```python
from build123d import *

# Parameters (mm, degrees)
SKETCH1_W           = 12.7
SKETCH1_H           = 152.4
BOSS_EXTRUDE1_DEPTH = 25.4
SKETCH6_W           = 50.8
SKETCH6_H           = 25.4
BOSS_EXTRUDE5_DEPTH = 2.54
SKETCH7_W           = 2.54
SKETCH7_H           = 25.4
BOSS_EXTRUDE6_DEPTH = 25.4


with BuildPart() as part:
    # Sketch1 → Boss-Extrude1 (new body)
    with BuildSketch(Plane(origin=(0, 0, 0), x_dir=(1, 0, 0), z_dir=(0, 1, 0))):
        with Locations((6.35, 76.2)):
            Rectangle(SKETCH1_W, SKETCH1_H)
    boss_extrude1 = extrude(amount=BOSS_EXTRUDE1_DEPTH)

    # Sketch6 → Boss-Extrude5 (add)
    with BuildSketch(Plane(origin=(12.7, 0, 0), x_dir=(0, 0, -1), z_dir=(1, 0, 0))):
        with Locations((127, 12.7)):
            Rectangle(SKETCH6_W, SKETCH6_H)
    boss_extrude5 = extrude(amount=BOSS_EXTRUDE5_DEPTH)

    # Sketch7 → Boss-Extrude6 (add)
    with BuildSketch(Plane(origin=(0, 25.4, 0), x_dir=(1, 0, 0), z_dir=(0, 1, 0))):
        with Locations((13.97, 127)):
            Rectangle(SKETCH7_W, SKETCH7_H)
    boss_extrude6 = extrude(amount=BOSS_EXTRUDE6_DEPTH)

    # Mirror1: Boss-Extrude1, Boss-Extrude5, Boss-Extrude6 across plane
    add(boss_extrude1.mirror(Plane(origin=(0, 25.4, 0), x_dir=(0, 0, 1), z_dir=(1, 0, 0))))
    add(boss_extrude5.mirror(Plane(origin=(0, 25.4, 0), x_dir=(0, 0, 1), z_dir=(1, 0, 0))))
    add(boss_extrude6.mirror(Plane(origin=(0, 25.4, 0), x_dir=(0, 0, 1), z_dir=(1, 0, 0))))


solid = part.part
```
Verification items for the finished model (mm, model axes). A direction names the side the tool comes from. Round coordinates to 2 decimals unless told otherwise and drop trailing zeros. Write each loop counter-clockwise with the first axis right and the second up, starting at its lowest first coordinate (ties: lowest second). Pieces come first, ordered by that corner, then holes.
1. Section check C-C on y = 16.5. Enter the section's corners in (x, z), plus the area to 3 significant figures.
2. Section check B-B on z = -122. Enter the section's corners in (x, y), plus the area to 3 significant figures.
3. Access from +Z, -Z, +X, -X, +Y, -Y to the whole of each face (thin tool, end or side, straight path). Record for faces 1 (the flat face through (14, 13, -101.6)), 2 (the flat face through (-12.7, 13, -50)), 3 (the flat face through (-14, 38, -139.7)), 4 (the flat face through (-14, 38, -114.3)).
4. Section check D-D on x = -7. Enter the section's corners in (y, z).
5. Draft check along X on faces 5 (the flat face through (12.7, 13, -50)), 6 (the flat face through (0, 13, 0)), 7 (the flat face through (12.7, 38, -127)). Enter one of: +X half, -X half, draft (parallel to the pull), parting line (faces both ways), or undercut.
6. Gauge pin test, flat ends, axial feed: P1, Ø1, axis at x = 5, y = 21.5, coming from the +Z side; P2, Ø1.3, axis at x = -14, y = 37.5, coming from the -Z side; P3, Ø1.3, axis at x = -14, y = 17, coming from the +Z side; P4, Ø4, axis at y = 19.5, z = -24.5, coming from the -X side. Record the tip position at first contact, or that the pin passes through.
7. Section check A-A on y = 40. Enter the section's corners in (x, z).
8. Scan lines: L1, parallel to X at y = 37, z = -122.5; L2, parallel to X at y = 23.5, z = -14.5; L3, parallel to Y at x = -3.5, z = -29. Record each from-to range of solid material in increasing order.
Answer:
1. outline: (-15.24, -152.4) - (15.24, -152.4) - (15.24, -101.6) - (12.7, -101.6) - (12.7, 0) - (-12.7, 0) - (-12.7, -101.6) - (-15.24, -101.6) - close
1. area: 4,130 mm2
2. outline: (-15.24, 0) - (15.24, 0) - (15.24, 50.8) - (12.7, 50.8) - (12.7, 25.4) - (-12.7, 25.4) - (-12.7, 50.8) - (-15.24, 50.8) - close
2. area: 903 mm2
3. face 1: +Z, +X, +Y, -Y
3. face 2: +Z, -X, +Y, -Y
3. face 3: -Z, +X, -X, +Y
3. face 4: +Z, +X, -X, +Y
4. outline: (0, -152.4) - (25.4, -152.4) - (25.4, 0) - (0, 0) - close
5. face 5: +X half
5. face 6: draft
5. face 7: undercut
6. P1: stops at z = 0
6. P2: stops at z = -139.7
6. P3: stops at z = -101.6
6. P4: stops at x = -12.7
7. outline: (-15.24, -139.7) - (-12.7, -139.7) - (-12.7, -114.3) - (-15.24, -114.3) - close; (12.7, -139.7) - (15.24, -139.7) - (15.24, -114.3) - (12.7, -114.3) - close
8. L1: x = -15.24 to -12.7, 12.7 to 15.24
8. L2: x = -12.7 to 12.7
8. L3: y = 0 to 25.4
